Could you check a few things on this drawing? It's one solid part, dimensions in mm from its lowest x, y, z. A direction names the side the tool comes from. Round coordinates to 2 decimals unless told otherwise and drop trailing zeros. Write each loop counter-clockwise with the first axis right and the second up, starting at its lowest first coordinate (ties: lowest second). Pieces come first, ordered by that corner, then holes. Notation, with made-up numbers: (38, 80.25) -> (96, 80.25) arc R21 cw to (96, 88.25) -> close; hole circle Ø1 at (50.5, 48.25). An arc over 180 degrees is marked (long way). Put each result on its own line as item: value. Start each with the question number.
1) I want a section at C-C, the plane y = 12.7. Give the number of separate pieces and of enclosed holes in the cut face.
2) Which directions (+Z, -Z, +X, -X, +Y, -Y) give clear straight access to the entire face, cutting with the end or side of a thin tool? Please do the marked faces 1 and 2.
3) If I drill on line 1 along Y through (x, z) = (0.9, 25.4) (1 decimal); line 2 along Y through (x, z) = (11, 26) (1 decimal); line 3 along Z through (x, y) = (12.7, 35.9) (1 decimal), over which ranges is the centre line in solid material (lowest first)? Write a range as [from, to].
4) I want a section at B-B, the plane z = 25.4. List the corners of the cut face in (x, y) for me (1 decimal), then the cut area to 3 significant figures.
5) I want a section at D-D, the plane z = 14.5. List the corners of the cut face in (x, y) for me (1 decimal).
6) I want a section at A-A, the plane x = 12.7. List the corners of the cut face in (y, z) for me (1 decimal).
7) Will these pins go through, and if not, where does the flat tip stop? P1, Ø4.5, axis at x = 12.7, z = 17.46, coming from the -Y side; P2, Ø17.5, axis at y = 26, z = 10.5, coming from the +X side (1 decimal).
8) We'd pull the mould along Z, two halves only. Please class the marked faces 3, 4 and 5: released by +Z, released by -Z, zero draft, split by the parting line, or undercut.
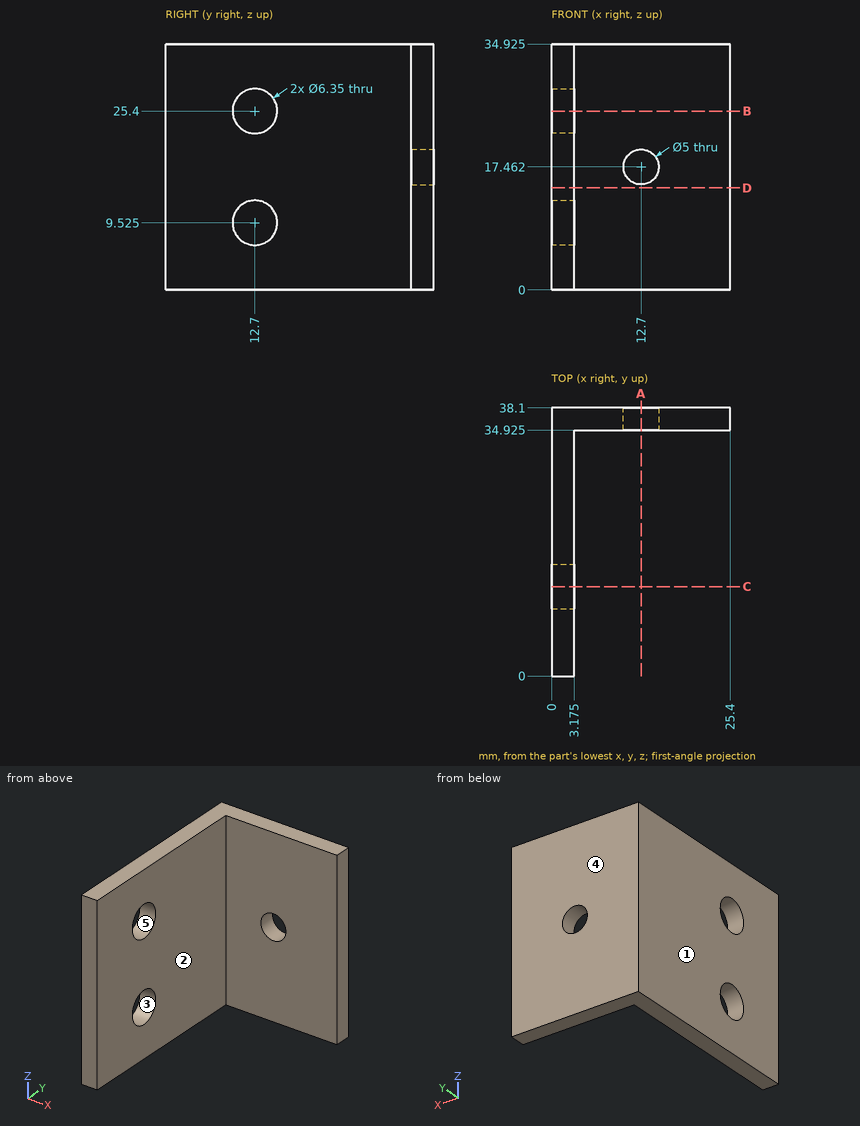
Findings:
1. separate pieces: 3
1. enclosed holes: 0
2. face 1: +Z, -Z, -X, +Y, -Y
2. face 2: +Z, -Z, +X, -Y
3. line 1: y = [0, 9.5], [15.9, 38.1]
3. line 2: y = [34.9, 38.1]
3. line 3: z = [0, 15], [20, 34.9]
4. outline: (0, 0) -> (3.2, 0) -> (3.2, 9.5) -> (0, 9.5) -> close; (0, 15.9) -> (3.2, 15.9) -> (3.2, 34.9) -> (25.4, 34.9) -> (25.4, 38.1) -> (0, 38.1) -> close
4. area: 171 mm2
5. outline: (0, 0) -> (3.2, 0) -> (3.2, 34.9) -> (25.4, 34.9) -> (25.4, 38.1) -> (0, 38.1) -> close
6. outline: (34.9, 0) -> (38.1, 0) -> (38.1, 15) -> (34.9, 15) -> close; (34.9, 20) -> (38.1, 20) -> (38.1, 34.9) -> (34.9, 34.9) -> close
7. P1: passes through
7. P2: stops at x = 3.2
8. face 3: undercut
8. face 4: zero draft
8. face 5: undercut
